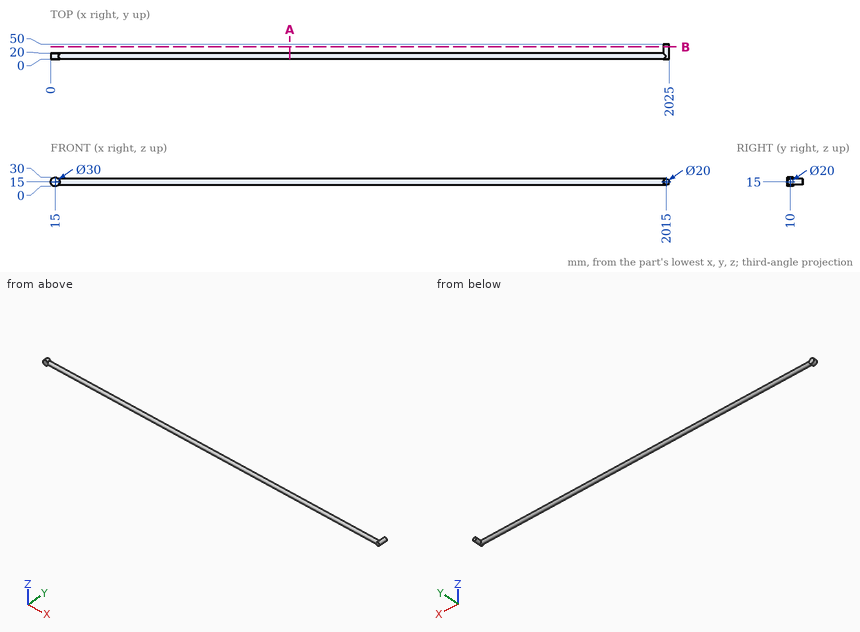
Design review of the part shown in the three views and the two pictorial views. Dimensions are in mm from the part's minimum x, y and z. Round coordinates to 2 decimals unless told otherwise and drop trailing zeros. Loops run counter-clockwise (first coordinate to the right, second up) from the corner with the lowest first, then second, coordinate; pieces in that order, holes last. Notation, with made-up numbers: M -19,55 L 32,55 A23 cw 32,77 Z; hole C 24.25,88.5 d6. An arc over 180 degrees is marked long. Answer as a JSON object with one key per item and string values.
Item 1: Clearance check with flat-ended pins moving along their axes: P1, Ø3, axis at y = 8, z = 22, coming from the -X side; P2, Ø5, axis at y = 15, z = 17.5, coming from the -X side; P3, Ø8, axis at x = 363.5, z = 3.5, coming from the -Y side; P4, Ø2, axis at x = 1242.5, z = 11, coming from the +Y side. State where each tip first meets the part, or that it passes through.
Answer sheet:
{"P1": "stops at x = 1.04", "P2": "stops at x = 0", "P3": "stops at y = 3.39", "P4": "stops at y = 19.54"}
Item 2: Wall thickness on L1, parallel to X at y = 11, z = 16; L2, parallel to X at y = 44.5, z = 14; L3, parallel to Y at x = 1888.5, z = 10.5: over which ranges is each line inside the solid? List them lowest first. Write a range as from..to.
Answer sheet:
{"L1": "x = 0.03..2024.95", "L2": "x = 2005.05..2024.95", "L3": "y = 1.07..18.93"}
Item 3: We need section A-A on x = 783.5. Give the boundary of the cut face in (y, z), and give its area (3 significant figures).
Answer sheet:
{"outline": "C 10,15 d20", "area": "314 mm^2"}
Item 4: We need section B-B on y = 40.5. Give the boundary of the cut face in (x, z).
Answer sheet:
{"outline": "C 2015,15 d20"}
